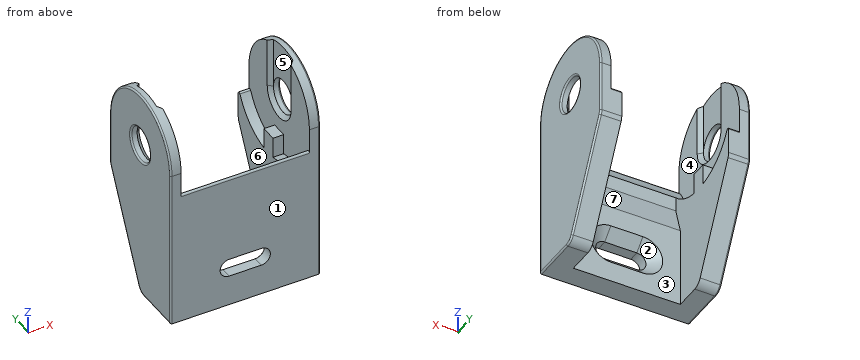
```python
from build123d import *

# Parameters (mm, degrees)
BOSS_EXTRUDE1_DEPTH = 14
SKETCH2_R           = 3.2
CUT_EXTRUDE1_DEPTH  = 48
CUT_EXTRUDE2_DEPTH  = 10
CUT_EXTRUDE4_DEPTH  = 12
FILLET1_R           = 0.3
CUT_EXTRUDE3_DEPTH  = 4
CHAMFER1_SIZE       = 2
FILLET2_R           = 2
FILLET3_R           = 0.3
SKETCH7_W           = 25.5
SKETCH7_H           = 10
CUT_EXTRUDE5_DEPTH  = 3.2
CHAMFER2_SIZE       = 0.75


with BuildPart() as part:
    # Sketch1 → Boss-Extrude1 (new, symmetric)
    with BuildSketch(Plane(origin=(0, 0, 0), x_dir=(0, 0, -1), z_dir=(1, 0, 0))):
        with BuildLine():
            Line((30, -10), (0, -10))
            ThreePointArc((0, -10), (-10, 0), (0, 10))
            Line((0, 10), (30, 10))
            Line((30, 10), (30, -10))
        make_face()
    extrude(amount=BOSS_EXTRUDE1_DEPTH, both=True)

    # Sketch2 → Cut-Extrude1 (cut)
    with BuildSketch(Plane(origin=(14, 0, 0), x_dir=(0, 0, -1), z_dir=(1, 0, 0))):
        Circle(SKETCH2_R)
        Polygon((30, 0), (10, 10), (30, 10), align=None)
    extrude(amount=-CUT_EXTRUDE1_DEPTH, mode=Mode.SUBTRACT)

    # Sketch4 → Cut-Extrude2 (cut, symmetric)
    with BuildSketch(Plane(origin=(0, 0, 0), x_dir=(0, 0, -1), z_dir=(1, 0, 0))):
        with BuildLine():
            Line((0, -10), (1.5, -10))
            Line((1.5, -10), (1.5, -7.5))
            Line((1.5, -7.5), (10, -7.5))
            Line((10, -7.5), (15, -6))
            Line((15, -6), (30, -6))
            Line((30, -6), (30, 0))
            Line((30, 0), (10, 10))
            Line((10, 10), (0, 10))
            ThreePointArc((0, 10), (-10, 0), (0, -10))
        make_face()
    extrude(amount=CUT_EXTRUDE2_DEPTH, both=True, mode=Mode.SUBTRACT)

    # Sketch6 → Cut-Extrude4 (cut, symmetric)
    with BuildSketch(Plane(origin=(0, 0, 0), x_dir=(0, 0, -1), z_dir=(1, 0, 0))):
        with BuildLine():
            Line((10.392304845, 1.5), (6.5, 1.5))
            Line((6.5, 1.5), (6.5, -1.5))
            Line((6.5, -1.5), (10.392304845, -1.5))
            ThreePointArc((10.392304845, -1.5), (-10.5, 0), (10.392304845, 1.5))
        make_face()
    extrude(amount=CUT_EXTRUDE4_DEPTH, both=True, mode=Mode.SUBTRACT)

    # Fillet1
    fillet1_edges = [part.edges().sort_by_distance(p)[0] for p in [
        (0, -10, -3.201562119),
        (-11, 10, -3.201562119),
        (11, 10, -3.201562119),
    ]]
    fillet(fillet1_edges, radius=FILLET1_R)

    # Sketch5 → Cut-Extrude3 (cut)
    with BuildSketch(Plane(origin=(0, -10, 0), x_dir=(1, 0, 0), z_dir=(0, 1, 0))):
        with BuildLine():
            Line((-3, 24.2), (3, 24.2))
            ThreePointArc((3, 24.2), (4.7, 22.5), (3, 20.8))
            Line((3, 20.8), (-3, 20.8))
            ThreePointArc((-3, 20.8), (-4.7, 22.5), (-3, 24.2))
        make_face()
    extrude(amount=CUT_EXTRUDE3_DEPTH, mode=Mode.SUBTRACT)

    # Chamfer1
    chamfer1_edges = [part.edges().sort_by_distance(p)[0] for p in [
        (0, -6, -24.2),
        (4.7, -6, -22.5),
        (0, -6, -20.8),
        (-4.7, -6, -22.5),
    ]]
    chamfer(chamfer1_edges, length=CHAMFER1_SIZE)

    # Fillet2
    fillet2_edges = [part.edges().sort_by_distance(p)[0] for p in [
        (-12, 0, -30),
        (-12, 10, -10),
        (12, 10, -10),
        (12, 0, -30),
    ]]
    fillet(fillet2_edges, radius=FILLET2_R)

    # Fillet3
    fillet3_edges = [part.edges().sort_by_distance(p)[0] for p in [
        (14, -5.618033989, -30),
        (-14, 5.170820393, -19.658359214),
        (-14, 10, -4.763932023),
        (-14, -0.184605753, -29.701301617),
        (-14, 9.946497979, -9.987369886),
        (14, 5.170820393, -19.658359214),
        (14, 10, -4.763932023),
        (14, -0.184605753, -29.701301617),
        (14, 9.946497979, -9.987369886),
        (-14, 0, 3.2),
        (14, 0, 3.2),
        (14, 0, 10),
        (-14, -5.618033989, -30),
        (-14, -10, -15),
        (-14, 0, 10),
        (14, -10, -15),
    ]]
    fillet(fillet3_edges, radius=FILLET3_R)

    # Sketch7 → Cut-Extrude5 (cut, symmetric)
    with BuildSketch(Plane(origin=(0, 0, 0), x_dir=(1, 0, 0), z_dir=(0, 1, 0))):
        with Locations((0, -5)):
            Rectangle(SKETCH7_W, SKETCH7_H)
    extrude(amount=CUT_EXTRUDE5_DEPTH, both=True, mode=Mode.SUBTRACT)

    # Chamfer2
    chamfer2_edges = [part.edges().sort_by_distance(p)[0] for p in [
        (12, 3.2, 4.737087713),
        (12, -3.2, 4.737087713),
        (12, -2.2627417, -2.2627417),
        (-12, 3.2, 4.737087713),
        (-12, -3.2, 4.737087713),
        (-12, 2.2627417, -2.2627417),
    ]]
    chamfer(chamfer2_edges, length=CHAMFER2_SIZE - 0.0001)  # a hair under: the kernel refuses the full size


solid = part.part
```
Model file for the job. Use its own axes, mm. Face numbers are marked on the shaded views. A direction names the side the tool comes from. Give positions to 0.01 mm unless a question says otherwise; leave off trailing zeros. Loops run counter-clockwise (first coordinate to the right, second up) from the corner with the lowest first, then second, coordinate; pieces in that order, holes last. Notation, with made-up numbers: (20.25, -29.75) -> (74.25, -29.75) arc R18 ccw to (74.25, -8.75) -> close; hole circle Ø11 at (16, -36). An arc over 180 degrees is marked (long way). Use CSV: the item, a comma, the result in double quotes. Start each with the question number.
1) Mould opens along Y. For the marked faces 5, 6 and 7 say: released by +Y, released by -Y, zero draft, split by the parting line, or undercut.
2) Slice it at A-A on x = -1.5. Give the cut face in (y, z).
3) Tool access for the marked faces 1, 2, 3 and 4: list every direction of +Z, -Z, +X, -X, +Y, -Y with a clear straight run to the whole face (end or side of a thin tool).
4) Slice it at B-B on y = -2.25. Give the number of separate pieces and of enclosed holes in the cut face, plus the area to 3 significant figures.
5) Flat gauge pins, fed straight in: pin 1 Ø1.3 at (x, z) = (0.5, -8.5) entering from +Y; pin 2 Ø8.5 at (y, z) = (0, 0) entering from +X; pin 3 Ø0.6 at (x, y) = (11, 0.5) entering from +Z; pin 4 Ø12 at (x, z) = (-2.5, -25.5) entering from +Y. Where does each tip first touch, or does it go through?
6) Wall check: line 1 (X direction, y = 4.75, z = 6); line 2 (X direction, y = -5.75, z = -11); line 3 (Y direction, x = -12.95, z = 0). Give the ranges that are in metal, low to high.
Computed values:
1,face 5,"undercut"
1,face 6,"zero draft"
1,face 7,"released by +Y"
2,outline,"(-10, -30) -> (-6, -30) -> (-6, -26.2) -> (-8, -24.2) -> (-10, -24.2) -> close; (-10, -20.8) -> (-8, -20.8) -> (-6, -18.8) -> (-6, -15) -> (-7.5, -10) -> (-7.5, -7.35) arc R10.5 cw to (-9.43, -4.62) arc R0.3 ccw to (-10, -4.75) -> close"
3,face 1,"+Z, -Z, +X, -X, -Y"
3,face 2,"+Y"
3,face 3,"+Z, -Z, +Y"
3,face 4,"+Z"
4,separate pieces,"4"
4,enclosed holes,"0"
4,area,"208 mm^2"
5,pin 1,"stops at y = -7.5"
5,pin 2,"stops at x = 14"
5,pin 3,"stops at z = -6.5"
5,pin 4,"stops at y = -6"
6,line 1,"x = -14 to -12, 12 to 14"
6,line 2,"x = -14 to -10, 10 to 14"
6,line 3,"y = -10 to -3.2, 3.2 to 10"
